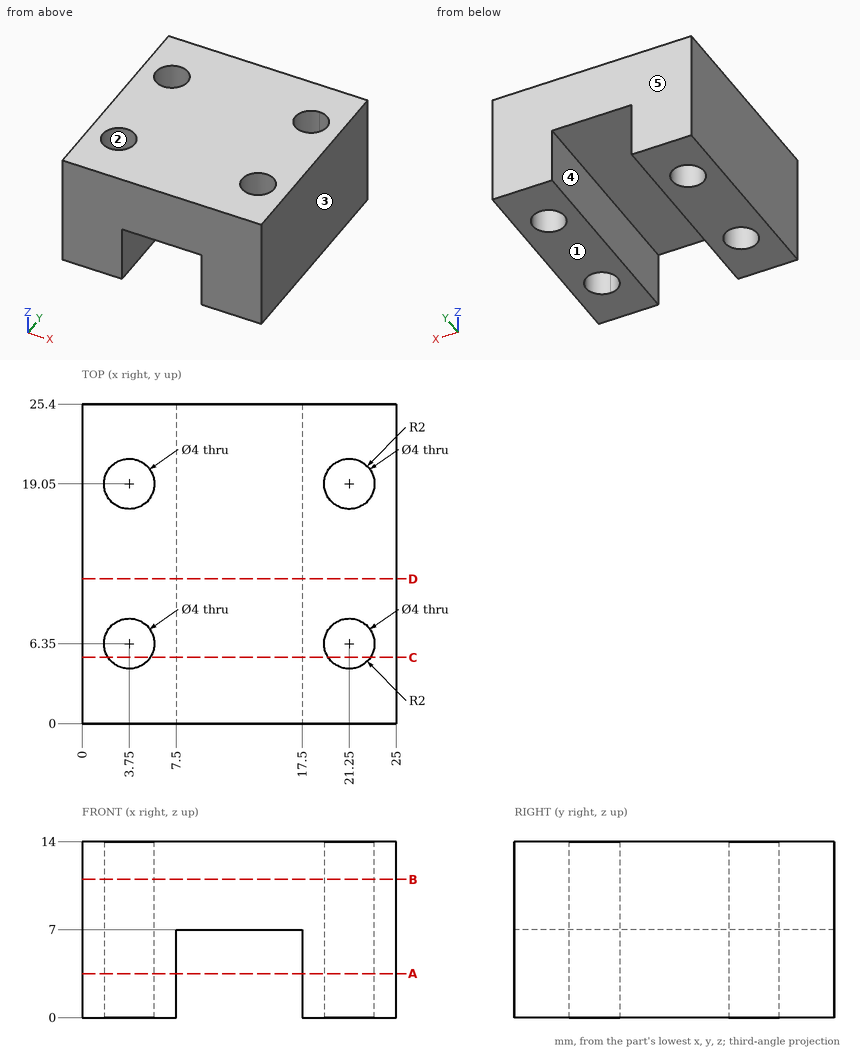
Geometry: see drawing. Coordinates: mm, zero at the bounding-box minimum. A direction names the side the tool comes from. Give positions to 0.01 mm unless a question says otherwise; leave off trailing zeros. Loops run counter-clockwise (first coordinate to the right, second up) from the corner with the lowest first, then second, coordinate; pieces in that order, holes last. Notation, with made-up numbers: (62.5, 60) -> (114.5, 60) arc R23 cw to (114.5, 71) -> close; hole circle Ø6 at (49.25, -22). An arc over 180 degrees is marked (long way). Answer as a JSON object with one key per item and string values. Group by question number.
Item 1: Reachability of the marked faces 4 and 5 from +Z, -Z, +X, -X, +Y, -Y: full face, straight path, thin tool, end or side. Return the list, or none.
Item 2: Cut plane A-A, the plane z = 3.5. Return the cut outline in (x, y), and give its area (3 significant figures).
Item 3: Line query: probe 1 along Y at (x, z) = (21.25, 11.25); probe 2 along X at (y, z) = (19.05, 7.75); probe 3 along X at (y, z) = (19.05, 5). Output: solid intervals per line, ascending.
Item 4: Pull-direction query (X, two-part tool) for the marked faces 1, 2 and 3; classes: released by +X, released by -X, zero draft, split by the parting line, or undercut.
Item 5: Cut plane C-C, the plane y = 5.25. Return the cut outline in (x, z).
Item 6: Cut plane B-B, the plane z = 11. Return the cut outline in (x, y).
Item 7: Cut plane D-D, the plane y = 11.5. Return the cut outline in (x, z), and give its area (3 significant figures).
Checks:
{
 "1": {"face 4": "-Z, +Y, -Y", "face 5": "+Z, -Z, +X, -X, +Y"},
 "2": {"outline": "(0, 0) -> (7.5, 0) -> (7.5, 25.4) -> (0, 25.4) -> close; (17.5, 0) -> (25, 0) -> (25, 25.4) -> (17.5, 25.4) -> close; hole circle Ø4 at (3.75, 6.35); hole circle Ø4 at (3.75, 19.05); hole (21.25, 4.35) arc R2 ccw to (23.25, 6.35) arc R2 ccw (long way) to start; hole (21.25, 21.05) arc R2 ccw (long way) to (23.25, 19.05) arc R2 ccw to start", "area": "331 mm²"},
 "3": {"probe 1": "y = 0 to 4.35, 8.35 to 17.05, 21.05 to 25.4", "probe 2": "x = 0 to 1.75, 5.75 to 19.25, 23.25 to 25", "probe 3": "x = 0 to 1.75, 5.75 to 7.5, 17.5 to 19.25, 23.25 to 25"},
 "4": {"face 1": "zero draft", "face 2": "undercut", "face 3": "released by +X"},
 "5": {"outline": "(0, 0) -> (2.08, 0) -> (2.08, 14) -> (0, 14) -> close; (5.42, 0) -> (7.5, 0) -> (7.5, 7) -> (17.5, 7) -> (17.5, 0) -> (19.58, 0) -> (19.58, 14) -> (5.42, 14) -> close; (22.92, 0) -> (25, 0) -> (25, 14) -> (22.92, 14) -> close"},
 "6": {"outline": "(0, 0) -> (25, 0) -> (25, 25.4) -> (0, 25.4) -> close; hole circle Ø4 at (3.75, 6.35); hole circle Ø4 at (3.75, 19.05); hole (21.25, 4.35) arc R2 ccw to (23.25, 6.35) arc R2 ccw (long way) to start; hole (21.25, 21.05) arc R2 ccw (long way) to (23.25, 19.05) arc R2 ccw to start"},
 "7": {"outline": "(0, 0) -> (7.5, 0) -> (7.5, 7) -> (17.5, 7) -> (17.5, 0) -> (25, 0) -> (25, 14) -> (0, 14) -> close", "area": "280 mm²"}
}
